from build123d import *

# Parameters (mm, degrees)
SKETCH1_R           = 3.5
BOSS_EXTRUDE1_DEPTH = 3
SKETCH2_R           = 2
BOSS_EXTRUDE2_DEPTH = 12
CHAMFER1_SIZE       = 0.3
CUT_EXTRUDE1_DEPTH  = 2


with BuildPart() as part:
    # Sketch1 → Boss-Extrude1 (new body)
    with BuildSketch(Plane.XY):
        Circle(SKETCH1_R)
    extrude(amount=BOSS_EXTRUDE1_DEPTH)

    # Sketch2 → Boss-Extrude2 (add)
    with BuildSketch(Plane(origin=(0, 0, 0), x_dir=(-1, 0, 0), z_dir=(0, 0, -1))):
        Circle(SKETCH2_R)
    extrude(amount=BOSS_EXTRUDE2_DEPTH)

    # Chamfer1
    chamfer1_edges = [part.edges().sort_by_distance(p)[0] for p in [
        (2, 0, -12),
    ]]
    chamfer(chamfer1_edges, length=CHAMFER1_SIZE)

    # Sketch3 → Cut-Extrude1 (cut)
    with BuildSketch(Plane.XY.offset(3)):
        Polygon((0, 1.732050808), (-1.5, 0.866025404), (-1.5, -0.866025404), (0, -1.732050808), (1.5, -0.866025404), (1.5, 0.866025404), align=None)
    extrude(amount=-CUT_EXTRUDE1_DEPTH, mode=Mode.SUBTRACT)


solid = part.part
Geometry check sheet. Reference: the model listing, model coordinates, mm. A direction names the side the tool comes from. Round coordinates to 2 decimals unless told otherwise and drop trailing zeros. Order: outer loops, then holes, each group sorted by start corner. A loop starts at its lowest first (then second) coordinate and runs counter-clockwise, first axis right, second up. Notation, with made-up numbers: M 33.25,17 L 39.25,17 A10 ccw 39.25,22 Z; hole C 4.25,82 d3. An arc over 180 degrees is marked long. Write each question's results on one line, items separated by ' | '. Start each with the question number.
1. Cross-section at B-B on z = -4. Record the boundary of the cut face in (x, y).
2. Cross-section at C-C on x = 2.5. Record the boundary of the cut face in (y, z).
3. Set-up check for faces 4 (the face through (-0.76, -1.293, 2.014)), 5 (the face through (2, -2, 0)), 6 (the face through (3.233, -1.341, 1.479)): record each of +Z, -Z, +X, -X, +Y, -Y from which the full face is reachable in a straight line by a thin tool's end or side.
4. Draft check along Y on faces 1 (the face through (-0.74, 1.305, 2.014)), 2 (the face through (2, 0, 3)), 3 (the face through (0, -2, -6)). Enter one of: pulls with the +Y half, pulls with the -Y half, needs draft (parallel to the pull), parting line crosses it, or undercut.
5. Material ranges on L1, parallel to Z at x = 0.75, y = -3; L2, parallel to X at y = 1, z = -9; L3, parallel to Y at x = 0, z = -7, recorded low to high. Write a range as from..to.
6. Go/stop test with flat-tipped pins: P1, Ø3, axis at y = -0.5, z = -2.5, coming from the -X side; P2, Ø2.5, axis at x = -0.5, y = 0, coming from the +Z side; P3, Ø1, axis at x = -0.5, z = -7.5, coming from the -Y side. Record where each tip stops, or that it passes through.
7. Cross-section at A-A on y = 0. Record the boundary of the cut face in (x, z).
8. Cross-section at D-D on y = 2.75. Record the boundary of the cut face in (x, z), plus the area to 3 significant figures.
Resolved:
1) outline: C 0,0 d4
2) outline: M -2.45,0 L 2.45,0 L 2.45,3 L -2.45,3 Z
3) face 4: +Z | face 5: -Z | face 6: +Z, -Z
4) face 1: undercut | face 2: needs draft | face 3: parting line crosses it
5) L1: 0..3 | L2: -1.73..1.73 | L3: -2..2
6) P1: x = -2 | P2: z = 3 | P3: y = -2
7) outline: M -3.5,0 L -2,0 L -2,-11.7 L -1.7,-12 L 1.7,-12 L 2,-11.7 L 2,0 L 3.5,0 L 3.5,3 L 1.5,3 L 1.5,1 L -1.5,1 L -1.5,3 L -3.5,3 Z
8) outline: M -2.17,0 L 2.17,0 L 2.17,3 L -2.17,3 Z | area: 13.0 mm2
